Design review of the part built by this model. Coordinates are the model's own, in mm. Face numbers are marked on the shaded views. A direction names the side the tool comes from. Coordinates: 2 decimals unless noted, no trailing zeros. Loops run counter-clockwise (first coordinate to the right, second up) from the corner with the lowest first, then second, coordinate; pieces in that order, holes last. Notation, with made-up numbers: M 76,14.25 L 81,14.25 A23 cw 81,33.25 Z; hole C 60.5,-22 d11. An arc over 180 degrees is marked long. Put each result on its own line as item: value. Start each with the question number.
(1) Clearance check with flat-ended pins moving along their axes: pin 1 (1.5 mm diameter, centred on x = 11.5, z = 7, fed in from +Y); pin 2 (3.5 mm diameter, centred on x = -7.5, y = -5, fed in from -Z). State where each tip first meets the part, or that it passes through.
(2) The part is to be moulded in two halves that separate along Y. For the marked faces 1, 2 and 3, say which applies: +Y half, -Y half, draft (parallel to the pull), parting line (faces both ways), or undercut.
(3) Take a section at A-A, the plane z = -17. Give the boundary of the cut face in (x, y).
(4) For probe 1 along Y at (x, z) = (7.5, -13.75); probe 2 along Z at (x, y) = (7.75, -5.25); probe 3 along Z at (x, y) = (-11.5, -6.75), list the stretches that pass through material, from the lowest coordinate up. Write a range as [from, to].
(5) For the marked faces 4 and 5, list the 3-axis set-ups (+Z, -Z, +X, -X, +Y, -Y) from which the entire face can be reached by the end or side of a thin tool; tool diameter is ignored.
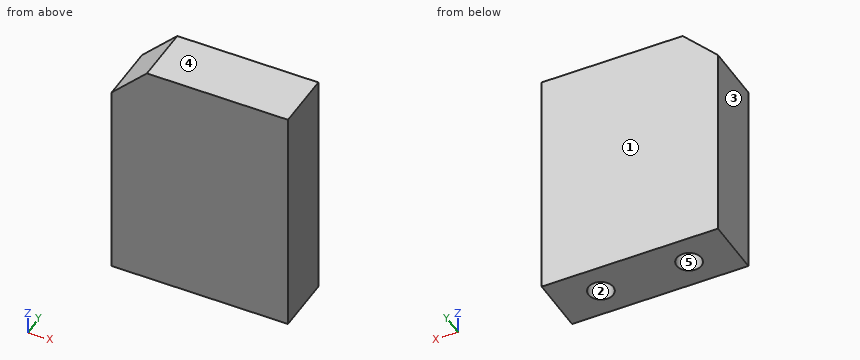
```python
from build123d import *

# Parameters (mm, degrees)
F0_W     = 30
F0_H     = 40
F1_DEPTH = 10
F2_SIZE  = 6
F4_D     = 4.2
F4_DEPTH = 14
F4_TIP   = 1.2618073


with BuildPart() as f1:
    # F0 (on Front) → F1 (new body)
    with BuildSketch(Plane.XZ):
        Rectangle(F0_W, F0_H)
    extrude(amount=F1_DEPTH)

    # F2
    f2_edges = [f1.edges().sort_by_distance(p)[0] for p in [
        (-15, -5, 20),
    ]]
    chamfer(f2_edges, length=F2_SIZE)

    # F4
    with Locations(Plane(origin=(0, 0, -20), x_dir=(1, 0, 0), z_dir=(0, 0, -1))):
        with Locations((7.5, 5), (-7.5, 5)):
            Hole(F4_D / 2, depth=F4_DEPTH)
            with Locations((0, 0, -(F4_DEPTH + F4_TIP / 2))):  # 118° drill point
                Cone(0, F4_D / 2, F4_TIP, mode=Mode.SUBTRACT)


solid = f1.part
```
Computed values:
1. pin 1: stops at y = 0
1. pin 2: stops at z = -5.79
2. face 1: +Y half
2. face 2: undercut
2. face 3: draft
3. outline: M -15,-10 L 15,-10 L 15,0 L -15,0 Z; hole C -7.5,-5 d4.2; hole C 7.5,-5 d4.2
4. probe 1: y = [-10, -7.1], [-2.9, 0]
4. probe 2: z = [-4.95, 20]
4. probe 3: z = [-20, 17.5]
5. face 4: +Z, +X, -X, +Y, -Y
5. face 5: -Z
